Here's how the part is built. I have some questions about the finished solid (model axes, mm). Face numbers are marked on the shaded views. A direction names the side the tool comes from. Coordinates: 2 decimals unless noted, no trailing zeros. Write each loop counter-clockwise with the first axis right and the second up, starting at its lowest first coordinate (ties: lowest second). Pieces come first, ordered by that corner, then holes.
Item 1: If we section it at C-C (z = 6.25): Count the separate pieces of the cut face and the enclosed holes in it, then the cut area to 3 significant figures.
Item 2: We'd pull the mould along Y, two halves only. Please class the marked faces 1, 2 and 3: +Y half, -Y half, draft (parallel to the pull), parting line (faces both ways), or undercut.
Item 3: I'm going to push flat-ended pins straight in: pin 1 Ø6 at (x, y) = (-7.5, 50.5) entering from +Z; pin 2 Ø1.5 at (y, z) = (35, 4) entering from +X; pin 3 Ø3 at (x, z) = (-7.5, 9) entering from +Y. Where does each tip first touch, or does it pass through?
Item 4: If we section it at A-A (y = 3): Please give me the cut outline in (x, z).
Item 5: For the marked faces 4, 5 and 6, which set-ups out of +Z, -Z, +X, -X, +Y, -Y let a thin tool reach every point of the face, with its end or its side?
Item 6: If we section it at B-B (y = 34): Please give me the cut outline in (x, z), then the cut area to 3 significant figures.
Item 7: If I drill on line 1 (Z direction, x = -7.5, y = 32.25); line 2 (Y direction, x = -2.5, z = 8) (3 decimals); line 3 (Y direction, x = -9, z = 3.75), over which ranges is the centre line in solid material (lowest first)?
from build123d import *

# Parameters (mm, degrees)
SKETCH1_W                     = 15
SKETCH1_H                     = 100
BOSS_EXTRUDE1_DEPTH           = 1
FILLET1_R                     = 7.5
BOSS_EXTRUDE2_DEPTH           = 10
BOSS_EXTRUDE2_DRAFT           = 16
SKETCH3_W                     = 15
SKETCH3_H                     = 22
BOSS_EXTRUDE2_PROFILE_2_DEPTH = 10
BOSS_EXTRUDE2_PROFILE_2_DRAFT = 16
SKETCH3_H_2                   = 31
BOSS_EXTRUDE2_PROFILE_3_DEPTH = 10
BOSS_EXTRUDE2_PROFILE_3_DRAFT = 16
SKETCH3_3_W                   = 15
SKETCH3_3_H                   = 17
BOSS_EXTRUDE3_DEPTH           = 10
CUT_EXTRUDE1_DEPTH            = 102.71528892
SKETCH5_R                     = 1
CUT_EXTRUDE2_DEPTH            = 95
FILLET2_R                     = 2
SKETCH6_R                     = 1.5
CUT_EXTRUDE3_DEPTH            = 102.71528892


with BuildPart() as part:
    # Sketch1 → Boss-Extrude1 (new body)
    with BuildSketch(Plane.XY):
        with Locations((-7.5, 50)):
            Rectangle(SKETCH1_W, SKETCH1_H)
    extrude(amount=BOSS_EXTRUDE1_DEPTH)

    # Fillet1
    fillet1_edges = [part.edges().sort_by_distance(p)[0] for p in [
        (0, 100, 0.5),
        (-15, 100, 0.5),
    ]]
    fillet(fillet1_edges, radius=FILLET1_R - 0.0001)  # a hair under: the kernel refuses the full size


with BuildPart() as boss_extrude2_tool:
    # Sketch3 → Boss-Extrude2 (with draft: the straight prism first)
    with BuildSketch(Plane.XY.offset(1)):
        with BuildLine():
            ThreePointArc((-7.5, 100), (-12.803300859, 97.803300859), (-15, 92.5))
            Line((-15, 92.5), (-15, 73))
            Line((-15, 73), (0, 73))
            Line((0, 73), (0, 92.5))
            ThreePointArc((0, 92.5), (-2.196699141, 97.803300859), (-7.5, 100))
        make_face()
    extrude(amount=BOSS_EXTRUDE2_DEPTH)
    # Boss-Extrude2: the draft: its side faces are tilted about the plane it starts from
    boss_extrude2_sides = [boss_extrude2_tool.faces().sort_by_distance(p)[0] for p in [
        (-7.5, 100, 6),
        (-7.5, 73, 6),
        (0, 82.75, 6),
        (-15, 82.75, 6),
    ]]
    draft(boss_extrude2_sides, Plane.XY.offset(1), BOSS_EXTRUDE2_DRAFT)


with BuildPart() as part_1:
    add(part.part)

    # Boss-Extrude2: add boss_extrude2_tool
    add(boss_extrude2_tool.part)


with BuildPart() as boss_extrude2_profile_2_tool:
    # Sketch3 → Boss-Extrude2 profile 2 (with draft: the straight prism first)
    with BuildSketch(Plane.XY.offset(1)):
        with Locations((-7.5, 61)):
            Rectangle(SKETCH3_W, SKETCH3_H)
    extrude(amount=BOSS_EXTRUDE2_PROFILE_2_DEPTH)
    # Boss-Extrude2 profile 2: the draft: its side faces are tilted about the plane it starts from
    boss_extrude2_profile_2_sides = [boss_extrude2_profile_2_tool.faces().sort_by_distance(p)[0] for p in [
        (-7.5, 72, 6),
        (-15, 61, 6),
        (-7.5, 50, 6),
        (0, 61, 6),
    ]]
    draft(boss_extrude2_profile_2_sides, Plane.XY.offset(1), BOSS_EXTRUDE2_PROFILE_2_DRAFT)


with BuildPart() as part_2:
    add(part_1.part)

    # Boss-Extrude2 profile 2: add boss_extrude2_profile_2_tool
    add(boss_extrude2_profile_2_tool.part)


with BuildPart() as boss_extrude2_profile_3_tool:
    # Sketch3 → Boss-Extrude2 profile 3 (with draft: the straight prism first)
    with BuildSketch(Plane.XY.offset(1)):
        with Locations((-7.5, 33.5)):
            Rectangle(SKETCH3_W, SKETCH3_H_2)
    extrude(amount=BOSS_EXTRUDE2_PROFILE_3_DEPTH)
    # Boss-Extrude2 profile 3: the draft: its side faces are tilted about the plane it starts from
    boss_extrude2_profile_3_sides = [boss_extrude2_profile_3_tool.faces().sort_by_distance(p)[0] for p in [
        (-7.5, 18, 6),
        (0, 33.5, 6),
        (-7.5, 49, 6),
        (-15, 33.5, 6),
    ]]
    draft(boss_extrude2_profile_3_sides, Plane.XY.offset(1), BOSS_EXTRUDE2_PROFILE_3_DRAFT)


with BuildPart() as part_3:
    add(part_2.part)

    # Boss-Extrude2 profile 3: add boss_extrude2_profile_3_tool
    add(boss_extrude2_profile_3_tool.part)

    # Sketch3<3> → Boss-Extrude3 (add)
    with BuildSketch(Plane.XY.offset(1)):
        with Locations((-7.5, 8.5)):
            Rectangle(SKETCH3_3_W, SKETCH3_3_H)
    extrude(amount=BOSS_EXTRUDE3_DEPTH)

    # Sketch4 → Cut-Extrude1 (cut, through all)
    with BuildSketch(Plane(origin=(0, 0, 0), x_dir=(0, 0, -1), z_dir=(1, 0, 0))):
        Polygon((-14.618204018, 86.618204018), (-1, 73), (-1, 72), (-12, 61), (-1, 50), (-1, 49), (-14.71384308, 35.28615692), (-14.71384308, 31.71384308), (-1, 18), (-1, 17), (-14.311925723, 3.688074277), (-29.385419391, 3.688074277), (-29.385419391, 86.618204018), align=None)
    extrude(amount=-CUT_EXTRUDE1_DEPTH, mode=Mode.SUBTRACT)

    # Sketch5 → Cut-Extrude2 (cut)
    with BuildSketch(Plane.XZ):
        with Locations(Location((-7.5, 9, 0), (0, 0, 270))):
            Circle(SKETCH5_R)
    extrude(amount=-CUT_EXTRUDE2_DEPTH, mode=Mode.SUBTRACT)

    # Fillet2
    fillet2_edges = [part_3.edges().sort_by_distance(p)[0] for p in [
        (-15, 12, 6),
        (0, 12, 6),
        (-12.132546142, 87.75, 11),
        (-7.5, 97.132546142, 11),
        (-7.5, 7, 11),
        (-12.132546142, 33.5, 11),
        (-2.867453858, 33.5, 11),
        (-7.5, 28, 11),
        (-7.5, 39, 11),
        (-12.132546142, 61, 11),
        (-2.867453858, 61, 11),
        (-7.5, 60, 11),
        (-7.5, 62, 11),
        (-2.867453858, 87.75, 11),
        (-7.5, 83, 11),
        (-13.566273071, 78, 6),
        (-1.433726929, 78, 6),
        (-13.566273071, 67, 6),
        (-1.433726929, 67, 6),
        (-13.566273071, 55, 6),
        (-1.433726929, 55, 6),
        (-13.566273071, 44, 6),
        (-1.433726929, 44, 6),
        (-13.566273071, 23, 6),
        (-1.433726929, 23, 6),
    ]]
    fillet(fillet2_edges, radius=FILLET2_R)

    # Sketch6 → Cut-Extrude3 (cut, through all)
    with BuildSketch(Plane.XY.offset(11)):
        with Locations((-12, 3)):
            Circle(SKETCH6_R)
        with Locations((-3, 3)):
            Circle(SKETCH6_R)
    extrude(amount=-CUT_EXTRUDE3_DEPTH, mode=Mode.SUBTRACT)


solid = part_3.part
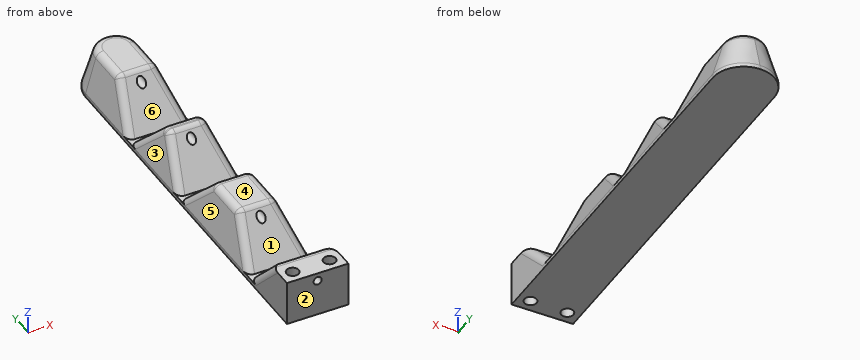
Answer list:
1. separate pieces: 4
1. enclosed holes: 2
1. area: 763 mm2
2. face 1: undercut
2. face 2: -Y half
2. face 3: draft
3. pin 1: stops at z = 4.5
3. pin 2: stops at x = -0.65
3. pin 3: stops at y = 98.14
4. outline: (-15, 0) - (-13.5, 0) - (-13.5, 11) - (-15, 11) - close; (-10.5, 0) - (-4.5, 0) - (-4.5, 11) - (-10.5, 11) - close; (-1.5, 0) - (0, 0) - (0, 11) - (-1.5, 11) - close; hole circle Ø2 at (-7.5, 9)
5. face 4: +Z, +X, -X, +Y, -Y
5. face 5: +Z, -X, +Y
5. face 6: +Z, +X, -X
6. outline: (-15, 0) - (0, 0) - (0, 1) - (-2.45, 9.55) arc R2 ccw to (-4.37, 11) - (-10.63, 11) arc R2 ccw to (-12.55, 9.55) - (-15, 1) - close; hole circle Ø2 at (-7.5, 9)
6. area: 132 mm2
7. line 1: z = 0 to 8, 10 to 11
7. line 2: y = 0 to 1.586, 4.414 to 10, 25.615 to 41.385, 57.615 to 64.385, 80.615 to 94.774
7. line 3: y = 0 to 14.25, 20.75 to 46.25, 52.75 to 69.25, 75.75 to 99.04
